Geometry check sheet. Reference: the model listing, model coordinates, mm. Face numbers are marked on the shaded views. A direction names the side the tool comes from. Give positions to 0.01 mm unless a question says otherwise; leave off trailing zeros. Loops run counter-clockwise (first coordinate to the right, second up) from the corner with the lowest first, then second, coordinate; pieces in that order, holes last. Notation, with made-up numbers: (-25.5, -17) -> (11.5, -17) arc R18 ccw to (11.5, 0) -> close; hole circle Ø11 at (-16, 18.5). An arc over 180 degrees is marked (long way). One line per item, written item: value. Start each with the question number.
(1) Scan lines: line 1 along Z through (x, y) = (10.5, -119); line 2 along Z through (x, y) = (-45.5, 206); line 3 along X through (y, z) = (106, 17.5). Record each from-to range of solid material in increasing order. Write a range as from..to.
(2) Gauge pin test, flat ends, axial feed: pin 1 Ø1 at (y, z) = (117.5, 22.5) entering from +X; pin 2 Ø4 at (x, y) = (7, -84.5) entering from +Z; pin 3 Ø1.5 at (y, z) = (77, 11.5) entering from +X. Record the tip position at first contact, or that the pin passes through.
(3) Tool access check on the marked faces 1 and 2. Record the directions out of +Z, -Z, +X, -X, +Y, -Y that give a thin tool (end or side, any length) a straight path to the whole face; none if there is none.
(4) Draft check along X on the marked faces 3, 4 and 5. Enter one of: pulls with the +X half, pulls with the -X half, needs draft (parallel to the pull), parting line crosses it, or undercut.
(5) Sectioned sample at B-B, the plane z = 15. Record the cut outline in (x, y), then the cut area to 3 significant figures.
(6) Sectioned sample at A-A, the plane y = -177.5. Record the cut outline in (x, z), then the cut area to 3 significant figures.
(7) Sectioned sample at C-C, the plane x = 20. Record the cut outline in (y, z).
from build123d import *

# Parameters (mm, degrees)
F1_DEPTH = 250


with BuildPart() as f1:
    # F0 (on Front) → F1 (new body, symmetric)
    with BuildSketch(Plane.XZ):
        with BuildLine():
            Line((-44.971709, 23.338451), (-68.018377, 4))
            Line((-68.018377, 4), (-68.018377, 0))
            Line((-68.018377, 0), (-44.971709, -13.306))
            ThreePointArc((-44.971709, -13.306), (8.098756, -5.765582), (61.265842, -12.5915))
            Line((61.265842, -12.5915), (83.074959, 0))
            Line((83.074959, 0), (83.074959, 4))
            Line((83.074959, 4), (60.028291, 23.338451))
            Line((60.028291, 23.338451), (30.028291, 23.338451))
            Line((30.028291, 23.338451), (30.028291, 22.038451))
            Line((30.028291, 22.038451), (-14.971709, 22.038451))
            Line((-14.971709, 22.038451), (-14.971709, 23.338451))
            Line((-14.971709, 23.338451), (-44.971709, 23.338451))
        make_face()
    extrude(amount=F1_DEPTH, both=True)


solid = f1.part
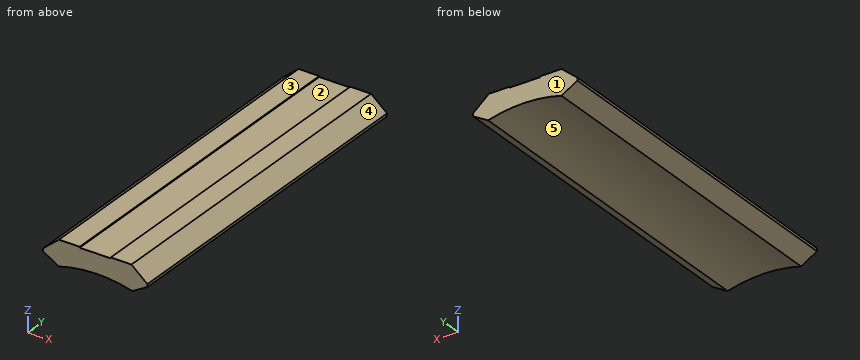
Calculated:
1. line 1: z = -5.76..22.04
1. line 2: z = -13..22.9
1. line 3: x = -51.93..66.99
2. pin 1: stops at x = 61.62
2. pin 2: stops at z = 22.04
2. pin 3: stops at x = 75.03
3. face 1: +Z, -Z, +X, -X, +Y
3. face 2: +Z, +Y, -Y
4. face 3: needs draft
4. face 4: pulls with the +X half
4. face 5: undercut
5. outline: (-54.91, -250) -> (69.97, -250) -> (69.97, 250) -> (-54.91, 250) -> close
5. area: 62,400 mm2
6. outline: (-68.02, 0) -> (-44.97, -13.31) arc R200 cw to (61.27, -12.59) -> (83.07, 0) -> (83.07, 4) -> (60.03, 23.34) -> (30.03, 23.34) -> (30.03, 22.04) -> (-14.97, 22.04) -> (-14.97, 23.34) -> (-44.97, 23.34) -> (-68.02, 4) -> close
6. area: 4,180 mm2
7. outline: (-250, -6.04) -> (250, -6.04) -> (250, 22.04) -> (-250, 22.04) -> close
